Here's how the part is built. I have some questions about the finished solid (model axes, mm). Round coordinates to 2 decimals unless told otherwise and drop trailing zeros. Write each loop counter-clockwise with the first axis right and the second up, starting at its lowest first coordinate (ties: lowest second). Pieces come first, ordered by that corner, then holes. Notation, with made-up numbers: (34, -37.5) - (60, -37.5) arc R9 cw to (60, -23.5) - close; hole circle Ø7 at (78.25, 51). An arc over 180 degrees is marked (long way). Return JSON: item names as keys, results as strings. Group by question number.
```python
from build123d import *

# Parameters (mm, degrees)
PLAT_W                          = 30
PLAT_H                          = 5
EL_MENT_M_CANO_SOUD_1_DEPTH     = 1850
DIAM_TRE_DU_PER_AGE_13_0_13_1_D = 13
R_P_TITION_LIN_AIRE2_COUNT      = 5
R_P_TITION_LIN_AIRE2_PITCH      = 432.5


with BuildPart() as part:
    # plat → Elément mécano-soudé1 (new body)
    with BuildSketch(Plane.YZ.offset(-925)):
        Rectangle(PLAT_W, PLAT_H)
    extrude(amount=EL_MENT_M_CANO_SOUD_1_DEPTH)

    # Diamètre du perçage Ø13.0 (13)1 (through all)
    with Locations(Plane(origin=(0, 0, -2.5), x_dir=(-1, 0, 0), z_dir=(0, 0, -1))):
        with Locations((865, 0)):
            diam_tre_du_per_age_13_0_13_1 = Hole(DIAM_TRE_DU_PER_AGE_13_0_13_1_D / 2)

    # Répétition linéaire2: Diamètre du perçage Ø13.0 (13)1 ×5
    with Locations(*[(i * R_P_TITION_LIN_AIRE2_PITCH, 0, 0) for i in range(1, R_P_TITION_LIN_AIRE2_COUNT)]):
        add(diam_tre_du_per_age_13_0_13_1, mode=Mode.SUBTRACT)


solid = part.part
```
1) Imagine slicing it at A-A (y = 0). Please give me the cut outline in (x, z), plus the area to 4 significant figures.
2) I need wall thicknesses on line 1 along X through (y, z) = (1.5, 1.1); line 2 along X through (y, z) = (0.25, 1.55); line 3 along Y through (x, z) = (-432.5, -1). Which ranges of each line are inside material? Lowest first, please.
3) Will these pins go through, and if not, where does the flat tip stop? pin 1 Ø17 at (x, y) = (0, 0) entering from +Z; pin 2 Ø8 at (x, y) = (865, 0) entering from -Z.
Results found:
{
 "1": {"outline": "(-925, -2.5) - (-871.5, -2.5) - (-871.5, 2.5) - (-925, 2.5) - close; (-858.5, -2.5) - (-439, -2.5) - (-439, 2.5) - (-858.5, 2.5) - close; (-426, -2.5) - (-6.5, -2.5) - (-6.5, 2.5) - (-426, 2.5) - close; (6.5, -2.5) - (426, -2.5) - (426, 2.5) - (6.5, 2.5) - close; (439, -2.5) - (858.5, -2.5) - (858.5, 2.5) - (439, 2.5) - close; (871.5, -2.5) - (925, -2.5) - (925, 2.5) - (871.5, 2.5) - close", "area": "8,925 mm²"},
 "2": {"line 1": "x = -925 to -871.32, -858.68 to -438.82, -426.18 to -6.32, 6.32 to 426.18, 438.82 to 858.68, 871.32 to 925", "line 2": "x = -925 to -871.5, -858.5 to -439, -426 to -6.5, 6.5 to 426, 439 to 858.5, 871.5 to 925", "line 3": "y = -15 to -6.5, 6.5 to 15"},
 "3": {"pin 1": "stops at z = 2.5", "pin 2": "passes through"}
}
